Check sheet for the drawn part. Datum: minimum x, y, z corner. Units: mm. Coordinates: 2 decimals unless noted, no trailing zeros. Write each loop counter-clockwise with the first axis right and the second up, starting at its lowest first coordinate (ties: lowest second). Pieces come first, ordered by that corner, then holes. Notation, with made-up numbers: (53, 22.5) -> (91, 22.5) arc R28 cw to (91, 57.5) -> close; hole circle Ø11 at (54.5, 46). An arc over 180 degrees is marked (long way). Answer in a Markdown table with one row per item. Add a question column.
Q1. Thickness scan on line 1 (X direction, y = 1.65, z = 62.5); line 2 (Z direction, x = 177.5, y = 2.65). Record the ranges inside material, lowest first.
Q2. Section check B-B, the plane x = 79. Record the boundary of the cut face in (y, z).
Q3. Gauge pin test, flat ends, axial feed: P1, Ø0.9, axis at y = 2, z = 63, coming from the -X side; P2, Ø0.9, axis at x = 180.5, y = 2, coming from the -Z side; P3, Ø0.9, axis at x = 171.5, y = 2, coming from the +Z side. Record the tip position at first contact, or that the pin passes through.
Q4. Section check A-A, the plane y = 1.95. Record the boundary of the cut face in (x, z).
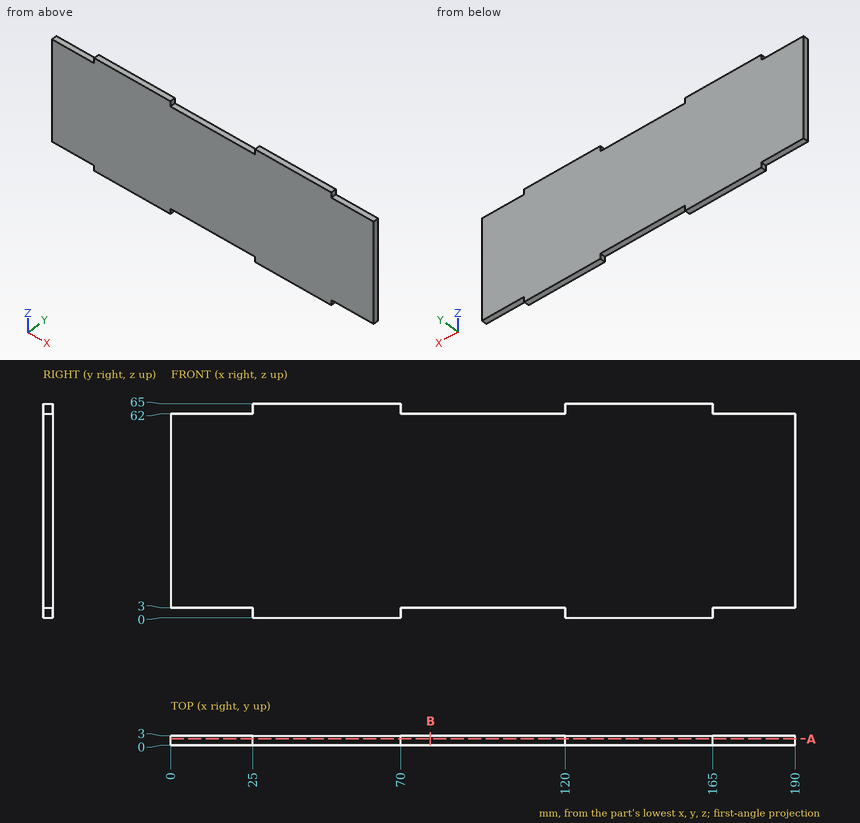
Calculated:
| question | item | result |
|---|---|---|
| 1 | line 1 | x = 25 to 70, 120 to 165 |
| 1 | line 2 | z = 3 to 62 |
| 2 | outline | (0, 3) -> (3, 3) -> (3, 62) -> (0, 62) -> close |
| 3 | P1 | stops at x = 25 |
| 3 | P2 | stops at z = 3 |
| 3 | P3 | stops at z = 62 |
| 4 | outline | (0, 3) -> (25, 3) -> (25, 0) -> (70, 0) -> (70, 3) -> (120, 3) -> (120, 0) -> (165, 0) -> (165, 3) -> (190, 3) -> (190, 62) -> (165, 62) -> (165, 65) -> (120, 65) -> (120, 62) -> (70, 62) -> (70, 65) -> (25, 65) -> (25, 62) -> (0, 62) -> close |
